```python
from build123d import *

# Parameters (mm, degrees)
F0_R     = 4
F1_DEPTH = 28
F2_SIZE  = 0.1
F3_R     = 4
F4_DEPTH = 6.5
F5_R     = 16.5
F6_DEPTH = 4
F7_R     = 1
F8_DEPTH = 4


with BuildPart() as f1:
    # F0 (on Front) → F1 (new body)
    with BuildSketch(Plane.XZ):
        Circle(F0_R)
    extrude(amount=-F1_DEPTH)

    # F2
    f2_edges = [f1.edges().sort_by_distance(p)[0] for p in [
        (-4, 0, 0),
    ]]
    chamfer(f2_edges, length=F2_SIZE)

    # F3 (on face) → F4 (join)
    with BuildSketch(Plane(origin=(0, 28, 0), x_dir=(-1, 0, 0), z_dir=(0, 1, 0))):
        Circle(F3_R)
    extrude(amount=F4_DEPTH)

    # F5 (on face) → F6 (join)
    with BuildSketch(Plane(origin=(0, 34.5, 0), x_dir=(-1, 0, 0), z_dir=(0, 1, 0))):
        Circle(F5_R)
    extrude(amount=F6_DEPTH)

    # F7 (on face) → F8 (join)
    with BuildSketch(Plane(origin=(0, 38.5, 0), x_dir=(-1, 0, 0), z_dir=(0, 1, 0))):
        with Locations((0, 13)):
            Circle(F7_R)
        with Locations((-13, 0)):
            Circle(F7_R)
        with Locations((0, -13)):
            Circle(F7_R)
        with Locations((13, 0)):
            Circle(F7_R)
    extrude(amount=F8_DEPTH)


solid = f1.part
```
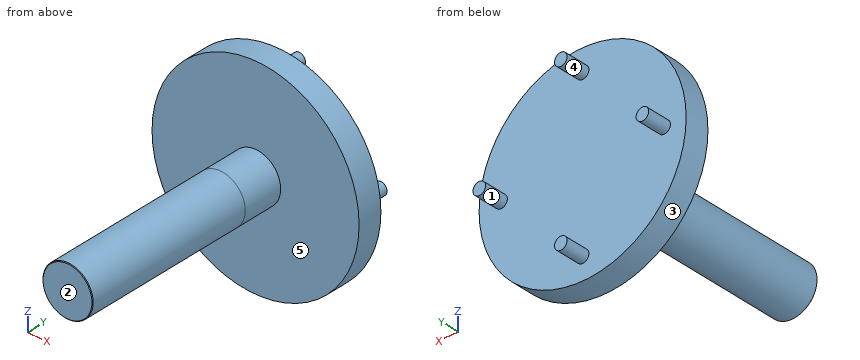
CAD build for the part. Positions are in the model's coordinates, mm. Face numbers are marked on the shaded views. A direction names the side the tool comes from. Give positions to 0.01 mm unless a question says otherwise; leave off trailing zeros. Loops run counter-clockwise (first coordinate to the right, second up) from the corner with the lowest first, then second, coordinate; pieces in that order, holes last. Notation, with made-up numbers: M 27,77 L 54,77 A22 cw 54,100 Z; hole C -34,-6.75 d8. An arc over 180 degrees is marked long. Use one line per item in the form item = value.
Item 1: Slice it at A-A (z = 0). List the corners of the cut face in (x, y), plus the area to 3 significant figures.
Determined:
outline = M -16.5,34.5 L -4,34.5 L -4,0.1 L -3.9,0 L 3.9,0 L 4,0.1 L 4,34.5 L 16.5,34.5 L 16.5,38.5 L 14,38.5 L 14,42.5 L 12,42.5 L 12,38.5 L -12,38.5 L -12,42.5 L -14,42.5 L -14,38.5 L -16.5,38.5 Z
area = 424 mm2
Item 2: Slice it at B-B (y = 24). List the corners of the cut face in (x, z).
Determined:
outline = C 0,0 d8
Item 3: Drill centre lines: probe 1 along Y at (x, z) = (2, 1); probe 2 along Y at (x, z) = (-8.5, 8); probe 3 along X at (y, z) = (5.5, 2). Where is each one in solid material? Low to high. Write a range as from..to.
Determined:
probe_1 = 0..38.5
probe_2 = 34.5..38.5
probe_3 = -3.46..3.46
Item 4: Flat gauge pins, fed straight in: pin 1 (8 mm diameter, centred on x = 13, z = 6, fed in from -Y); pin 2 (8 mm diameter, centred on y = 27, z = -3.5, fed in from +X); pin 3 (10 mm diameter, centred on x = 4.5, z = -7.5, fed in from +Y). Where does each tip first touch, or does it go through?
Determined:
pin_1 = 34.5
pin_2 = 4
pin_3 = 38.5
Item 5: Slice it at C-C (x = -13). List the corners of the cut face in (y, z), plus the area to 3 significant figures.
Determined:
outline = M 34.5,-10.16 L 38.5,-10.16 L 38.5,-1 L 42.5,-1 L 42.5,1 L 38.5,1 L 38.5,10.16 L 34.5,10.16 Z
area = 89.3 mm2
Item 6: Slice it at D-D (z = 13). List the corners of the cut face in (x, y).
Determined:
outline = M -10.16,34.5 L 10.16,34.5 L 10.16,38.5 L 1,38.5 L 1,42.5 L -1,42.5 L -1,38.5 L -10.16,38.5 Z
Item 7: Which spindle directions (+Z, -Z, +X, -X, +Y, -Y) get a long thin tool onto all of the face, cutting with end or side? Do the marked faces 1 and 2. Say none if no direction does.
Determined:
face_1 = +Y
face_2 = +Z, -Z, +X, -X, -Y
Item 8: Two-plate mould, pull along Z, no slides. Class the marked faces 3, 4 and 5: pulls with the +Z half, pulls with the -Z half, needs draft (parallel to the pull), parting line crosses it, or undercut.
Determined:
face_3 = parting line crosses it
face_4 = undercut
face_5 = needs draft
